The listing builds one solid part. Answer for the finished solid, in the listing's coordinates (mm). Face numbers are marked on the shaded views. Give positions to 0.01 mm unless a question says otherwise; leave off trailing zeros. Order: outer loops, then holes, each group sorted by start corner. A loop starts at its lowest first (then second) coordinate and runs counter-clockwise, first axis right, second up. Notation, with made-up numbers: (-38.5, 20.5) - (-3.5, 20.5) arc R12 ccw to (-3.5, 35.5) - close; hole circle Ø4 at (-22.5, -25). An arc over 180 degrees is marked (long way). Use a Markdown table: item, result. Add a question column.
1) Find section B-B, the plane y = 81. Determine the outline of the cut face in (x, z), plus the area to 3 significant figures.
2) Find section D-D, the plane z = -309.5. Determine the outline of the cut face in (x, y), plus the area to 3 significant figures.
3) Find section A-A, the plane x = 0. Determine the outline of the cut face in (y, z).
4) The mould has two halves that part along X. Classify the marked faces 1, 2 and 3: released by +X, released by -X, zero draft, split by the parting line, or undercut.
5) Straight lines are drawn through the part: line 1 (Z direction, x = -22, y = 80); line 2 (Z direction, x = 36, y = 45); line 3 (Y direction, x = 2, z = -61.5). For each, find the intervals that lie inside material, in ascending order.
6) Flat-ended cylindrical pins translate along their axes: pin 1 (3 mm diameter, centred on y = 71, z = -230, fed in from +X); pin 2 (2 mm diameter, centred on y = 87, z = -63.5, fed in from +X); pin 3 (6 mm diameter, centred on x = -11, z = -249.5, fed in from +Y). Find the tip coordinate at first contact, or state that the pin passes through.
7) Find section C-C, the plane z = -65.5. Determine the outline of the cut face in (x, y), plus the area to 3 significant figures.
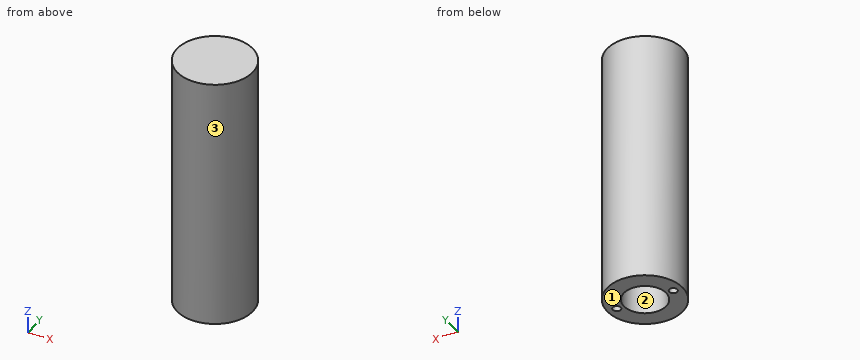
Autodesk Inventor part; units mm, degrees
ref_plane "YZ Plane" through (0, 0, 0) normal (1, 0, 0) x (0, 1, 0)
ref_plane "XZ Plane" through (0, 0, 0) normal (0, 1, 0) x (-1, 0, 0)
ref_plane "XY Plane" through (0, 0, 0) normal (0, 0, 1) x (1, 0, 0)
sketch "Sketch2" plane through (0, 0, 0) normal (1, 0, 0) x (0, 1, 0)
  line L0 (0, 0) -> (50, 0)
  line L1 (50, -335) -> (0, -335)
  line L2 (0, -335) -> (0, 0)
  line L3 (0, 0) -> (50, 0)
  line L4 (50, 0) -> (50, -26)
  line L5 (50, -26) -> (12.5, -26)
  line L6 (50, -335) -> (50, -248)
  line L7 (50, -248) -> (12.5, -248)
  line L8 (12.5, -26) -> (12.5, -248)
  line L9 (0, -335) -> (0, -465) construction
  dimension "d4" = 50
  dimension "d7" = 335
  dimension "d8" = 50
  dimension "d9" = 26
  dimension "d10" = 37.5
  dimension "d12" = 37.5
  dimension "d20" = 87
revolve "Revolution1" add sketch "Sketch2" angle 360 about axis through (0, 50, 0) along (0, 0, -1)
sketch "Sketch3" plane through (0, 50, -335) normal (0, 0, -1) x (-1, 0, 0)
  circle A0 centre (0, 0) radius 28
  point P0 (0, -50)
  dimension "d14" = 56
extrude "Extrusion2" cut sketch "Sketch3" against normal blind 309
sketch "Sketch4" plane through (0, 50, -335) normal (0, 0, -1) x (-1, 0, 0)
  circle A0 centre (0, 0) radius 37.5
  point P0 (0, -50)
  point P1 (37.5, 0)
  point P2 (-37.5, 0)
  dimension "d21" = 37.5
  dimension "d22" = 37.5
hole "Hole1" at (-37.5, 50, -335) at (37.5, 50, -335) direction (0, 0, 1) diameter 10.5918 depth 30 tip angle 137
equation "\"d4\" = d8"
equation "\"d12\" = d10"
properties part number "CilindroHidraulico_1"
The answers:
| question | item | result |
|---|---|---|
| 1 | outline | (-39.23, -335) - (39.23, -335) - (39.23, 0) - (-39.23, 0) - close; hole (-21.1, -248) - (21.1, -248) - (21.1, -26) - (-21.1, -26) - close |
| 1 | area | 16,900 mm2 |
| 2 | outline | circle Ø100 at (0, 50); hole circle Ø10.59 at (-37.5, 50); hole circle Ø56 at (0, 50); hole circle Ø10.59 at (37.5, 50) |
| 2 | area | 5,210 mm2 |
| 3 | outline | (0, -335) - (22, -335) - (22, -248) - (12.5, -248) - (12.5, -26) - (87.5, -26) - (87.5, -248) - (78, -248) - (78, -335) - (100, -335) - (100, 0) - (0, 0) - close |
| 4 | face 1 | zero draft |
| 4 | face 2 | undercut |
| 4 | face 3 | split by the parting line |
| 5 | line 1 | -335 to -248, -26 to 0 |
| 5 | line 2 | -304.97 to -248, -26 to 0 |
| 5 | line 3 | 0.04 to 12.55, 87.45 to 99.96 |
| 6 | pin 1 | x = 46.04 |
| 6 | pin 2 | x = 34.7 |
| 6 | pin 3 | y = 99.36 |
| 7 | outline | circle Ø100 at (0, 50); hole circle Ø75 at (0, 50) |
| 7 | area | 3,440 mm2 |
